Source: CAD feature listing. Evaluate the final solid. Frame: model axes, mm. Face numbers are marked on the shaded views. Round coordinates to 2 decimals unless told otherwise and drop trailing zeros. Loops run counter-clockwise (first coordinate to the right, second up) from the corner with the lowest first, then second, coordinate; pieces in that order, holes last. Notation, with made-up numbers: M 40.5,-1.75 L 78.5,-1.75 A35 ccw 78.5,32.25 Z; hole C -36,78 d5. An arc over 180 degrees is marked long. Answer as a JSON object with one key per item and string values.
from build123d import *

# Parameters (mm, degrees)
SKETCH1_R           = 62.5
BOSS_EXTRUDE1_DEPTH = 5
CUT_EXTRUDE1_START  = 55
SKETCH2_R           = 2
CUT_EXTRUDE1_DEPTH  = 10
CUT_EXTRUDE2_START  = -65
SKETCH2_2_R         = 2
CUT_EXTRUDE2_DEPTH  = 10
CUT_EXTRUDE3_START  = 55
SKETCH3_R           = 2
CUT_EXTRUDE3_DEPTH  = 10
CUT_EXTRUDE4_START  = -65
SKETCH3_2_R         = 2
CUT_EXTRUDE4_DEPTH  = 10
BOSS_EXTRUDE2_START = 10
BOSS_EXTRUDE2_DEPTH = 10
FILLET1_R           = 10
CUT_EXTRUDE5_START  = 60
SKETCH6_R           = 2
CUT_EXTRUDE5_DEPTH  = 10
CHAMFER1_SIZE       = 1


with BuildPart() as part:
    # Sketch1 → Boss-Extrude1 (new, symmetric)
    with BuildSketch(Plane.XY):
        Circle(SKETCH1_R)
    extrude(amount=BOSS_EXTRUDE1_DEPTH, both=True)

    # Sketch2 → Cut-Extrude1 (cut)
    with BuildSketch(Plane(origin=(0, 0, 0), x_dir=(1, 0, 0), z_dir=(0, 1, 0)).offset(CUT_EXTRUDE1_START)):
        with Locations(Location((0, 0, 0), (0, 0, 90))):
            Circle(SKETCH2_R)
    extrude(amount=CUT_EXTRUDE1_DEPTH, mode=Mode.SUBTRACT)

    # Sketch2<2> → Cut-Extrude2 (cut)
    with BuildSketch(Plane(origin=(0, 0, 0), x_dir=(1, 0, 0), z_dir=(0, 1, 0)).offset(CUT_EXTRUDE2_START)):
        with Locations(Location((0, 0, 0), (0, 0, 90))):
            Circle(SKETCH2_2_R)
    extrude(amount=CUT_EXTRUDE2_DEPTH, mode=Mode.SUBTRACT)

    # Sketch3 → Cut-Extrude3 (cut)
    with BuildSketch(Plane(origin=(0, 0, 0), x_dir=(0, 0, -1), z_dir=(1, 0, 0)).offset(CUT_EXTRUDE3_START)):
        Circle(SKETCH3_R)
    extrude(amount=CUT_EXTRUDE3_DEPTH, mode=Mode.SUBTRACT)

    # Sketch3<2> → Cut-Extrude4 (cut)
    with BuildSketch(Plane(origin=(0, 0, 0), x_dir=(0, 0, -1), z_dir=(1, 0, 0)).offset(CUT_EXTRUDE4_START)):
        Circle(SKETCH3_2_R)
    extrude(amount=CUT_EXTRUDE4_DEPTH, mode=Mode.SUBTRACT)

    # Sketch4 → Boss-Extrude2 (add)
    with BuildSketch(Plane.XY.offset(5).offset(BOSS_EXTRUDE2_START)):
        with BuildLine():
            Line((-31.25, 54.126587737), (-28.75, 49.796460718))
            ThreePointArc((-28.75, 49.796460718), (0, 57.5), (28.75, 49.796460718))
            Line((28.75, 49.796460718), (31.25, 54.126587737))
            ThreePointArc((31.25, 54.126587737), (0, 62.5), (-31.25, 54.126587737))
        make_face()
    extrude(amount=-BOSS_EXTRUDE2_DEPTH)

    # Fillet1
    fillet1_edges = [part.edges().sort_by_distance(p)[0] for p in [
        (-30, 51.961524227, 15),
        (30, 51.961524227, 15),
    ]]
    fillet(fillet1_edges, radius=FILLET1_R - 0.0001)  # a hair under: the kernel refuses the full size

    # Sketch6 → Cut-Extrude5 (cut)
    with BuildSketch(Plane(origin=(0, 0, 0), x_dir=(1, 0, 0), z_dir=(0, 1, 0)).offset(CUT_EXTRUDE5_START)):
        with Locations(Location((0, -10, 0), (0, 0, 90))):
            Circle(SKETCH6_R)
    extrude(amount=CUT_EXTRUDE5_DEPTH, mode=Mode.SUBTRACT)

    # Chamfer1
    chamfer1_edges = [part.edges().sort_by_distance(p)[0] for p in [
        (-62.5, 0, -5),
    ]]
    chamfer(chamfer1_edges, length=CHAMFER1_SIZE)


solid = part.part
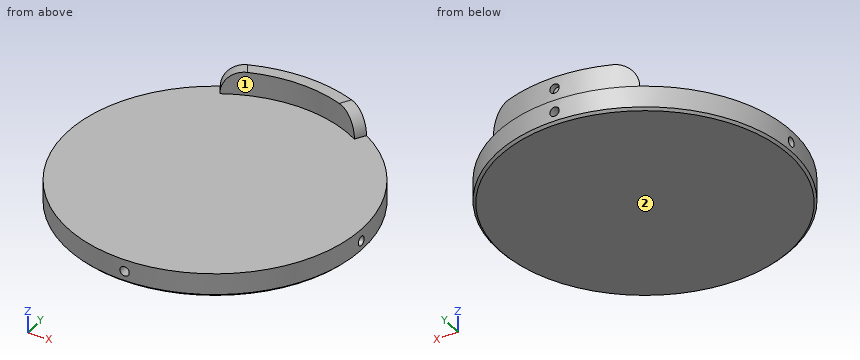
Item 1: Line query: probe 1 along Z at (x, y) = (-26, 23); probe 2 along Z at (x, y) = (58.75, 0); probe 3 along Y at (x, z) = (1, 1). Output: solid intervals per line, ascending. Write a range as from..to.
Answer sheet:
{"probe 1": "z = -5..5", "probe 2": "z = -5..-2, 2..5", "probe 3": "y = -55..55"}
Item 2: Section D-D on z = 10. Return the cut outline in (x, y), then the cut area to 3 significant figures.
Answer sheet:
{"outline": "M -30.08,54.78 L -27.58,50.45 A57.5 cw 27.58,50.45 L 30.08,54.78 A62.5 ccw 2,62.47 L 2,60 L -2,60 L -2,62.47 A62.5 ccw Z", "area": "291 mm²"}
Item 3: Section C-C on z = 0. Return the cut outline in (x, y).
Answer sheet:
{"outline": "M -62.47,-2 A62.5 ccw -2,-62.47 L -2,-55 L 2,-55 L 2,-62.47 A62.5 ccw 62.47,-2 L 55,-2 L 55,2 L 62.47,2 A62.5 ccw 2,62.47 L 2,55 L -2,55 L -2,62.47 A62.5 ccw -62.47,2 L -55,2 L -55,-2 Z"}
Item 4: Contact query for flat-ended pins moving along their axis: pin 1 Ø5 at (x, z) = (-27.5, 5.5) entering from +Y; pin 2 Ø3 at (x, z) = (-12, 4.5) entering from -Y; pin 3 Ø2.5 at (y, z) = (0, 0) entering from +X. Output: stop coordinate, or through.
Answer sheet:
{"pin 1": "stops at y = 57.28", "pin 2": "stops at y = -61.61", "pin 3": "stops at x = 55"}
Item 5: Pull-direction query (X, two-part tool) for the marked faces 1 and 2; classes: pulls with the +X half, pulls with the -X half, needs draft (parallel to the pull), parting line crosses it, or undercut.
Answer sheet:
{"face 1": "undercut", "face 2": "needs draft"}
Item 6: Section B-B on y = 0. Return the cut outline in (x, z), then the cut area to 3 significant figures.
Answer sheet:
{"outline": "M -62.5,-4 L -61.5,-5 L 61.5,-5 L 62.5,-4 L 62.5,-2 L 55,-2 L 55,2 L 62.5,2 L 62.5,5 L -62.5,5 L -62.5,2 L -55,2 L -55,-2 L -62.5,-2 Z", "area": "1,190 mm²"}
Item 7: Section A-A on x = 0. Return the cut outline in (y, z), then the cut area to 3 significant figures.
Answer sheet:
{"outline": "M -62.5,-4 L -61.5,-5 L 61.5,-5 L 62.5,-4 L 62.5,-2 L 55,-2 L 55,2 L 62.5,2 L 62.5,8 L 60,8 L 60,12 L 62.5,12 L 62.5,15 L 57.5,15 L 57.5,5 L -62.5,5 L -62.5,2 L -55,2 L -55,-2 L -62.5,-2 Z", "area": "1,230 mm²"}
